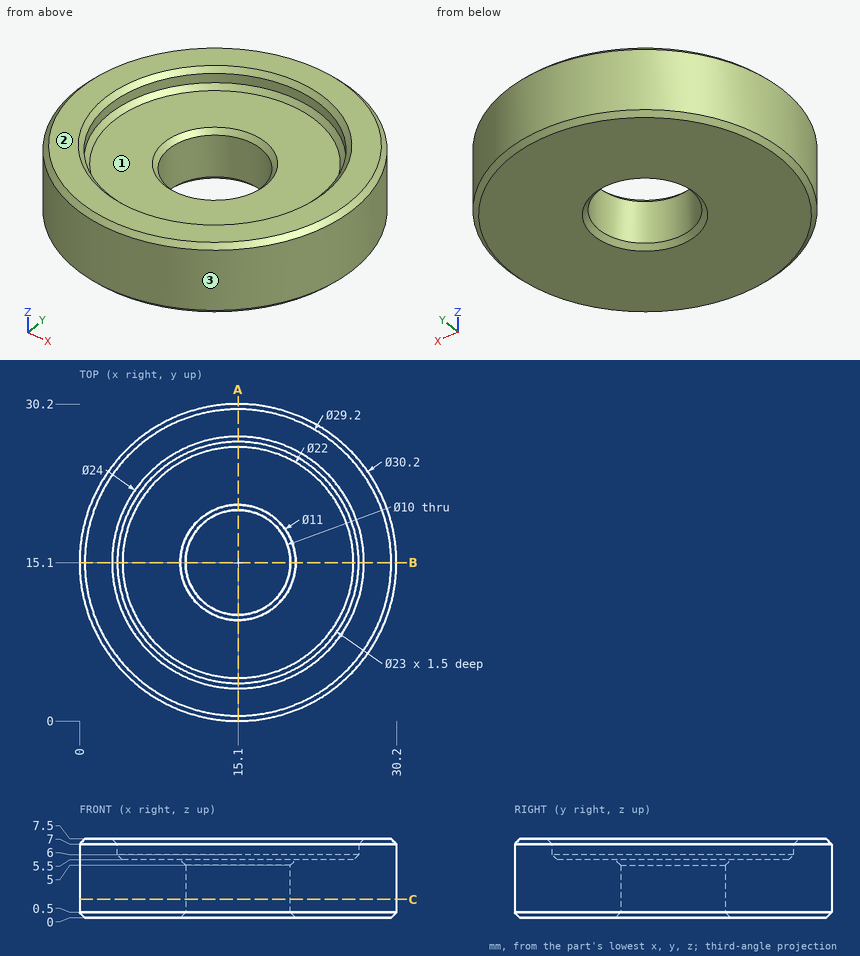
Verification items for this drawing (mm, ordinates from the low corner). Coordinates: 2 decimals unless noted, no trailing zeros. Loops run counter-clockwise (first coordinate to the right, second up) from the corner with the lowest first, then second, coordinate; pieces in that order, holes last. Notation, with made-up numbers: (-36, 87) -> (-15, 87) arc R23 cw to (-15, 122) -> close; hole circle Ø5 at (48, 84). An arc over 180 degrees is marked (long way). Put each result on its own line as item: value.
1. Mould release check, pull along X, two halves, no side actions. Record for the marked faces 1, 2 and 3: pulls with the +X half, pulls with the -X half, needs draft (parallel to the pull), parting line crosses it, or undercut.
Result set:
face 1: undercut
face 2: needs draft
face 3: parting line crosses it
2. Gauge pin test, flat ends, axial feed: P1, Ø1.5, axis at x = 10, z = 3.5, coming from the +Y side; P2, Ø6.5, axis at x = 17.5, y = 13, coming from the +Z side. Record the tip position at first contact, or that the pin passes through.
Result set:
P1: stops at y = 29.56
P2: stops at z = 5.5
3. Section check C-C, the plane z = 1.75. Record the boundary of the cut face in (x, y), then the cut area to 3 significant figures.
Result set:
outline: circle Ø30.2 at (15.1, 15.1); hole circle Ø10 at (15.1, 15.1)
area: 638 mm^2
4. Thickness scan on line 1 (Y direction, x = 15.1, z = 6.35); line 2 (Y direction, x = 15.1, z = 1.65); line 3 (Z direction, x = 22, y = 15). Record the ranges inside material, lowest first.
Result set:
line 1: y = 0 to 3.6, 26.6 to 30.2
line 2: y = 0 to 10.1, 20.1 to 30.2
line 3: z = 0 to 5.5
5. Section check A-A, the plane x = 15.1. Record the boundary of the cut face in (y, z).
Result set:
outline: (0, 0.5) -> (0.5, 0) -> (9.6, 0) -> (10.1, 0.5) -> (10.1, 5) -> (9.6, 5.5) -> (4.1, 5.5) -> (3.6, 6) -> (3.6, 7) -> (3.1, 7.5) -> (0.5, 7.5) -> (0, 7) -> close; (20.1, 0.5) -> (20.6, 0) -> (29.7, 0) -> (30.2, 0.5) -> (30.2, 7) -> (29.7, 7.5) -> (27.1, 7.5) -> (26.6, 7) -> (26.6, 6) -> (26.1, 5.5) -> (20.6, 5.5) -> (20.1, 5) -> close
